Geometry check sheet. Reference: the model listing, model coordinates, mm. A direction names the side the tool comes from. Coordinates: 2 decimals unless noted, no trailing zeros. Write each loop counter-clockwise with the first axis right and the second up, starting at its lowest first coordinate (ties: lowest second). Pieces come first, ordered by that corner, then holes. Notation, with made-up numbers: (-3.5, 70) - (18.5, 70) arc R21 cw to (18.5, 78) - close; hole circle Ø1 at (82.5, 45.5). An arc over 180 degrees is marked (long way). Answer as a JSON object with one key per item and string values. Group by question number.
from build123d import *

# Parameters (mm, degrees)
SKETCH1_W           = 20
SKETCH1_H           = 20
SKETCH1_R           = 6
BOSS_EXTRUDE1_DEPTH = 5


with BuildPart() as part:
    # Sketch1 → Boss-Extrude1 (new body)
    # profile 1 of 3: a face of its own
    with BuildSketch(Plane.XY):
        Rectangle(SKETCH1_W, SKETCH1_H)
        Circle(SKETCH1_R, mode=Mode.SUBTRACT)
    # profile 2 of 3: a face of its own
    with BuildSketch(Plane.XY):
        with BuildLine():
            ThreePointArc((3.31662479, 5), (0, 6), (-3.31662479, 5))
            Line((-3.31662479, 5), (3.31662479, 5))
        make_face()
    # profile 3 of 3: a face of its own
    with BuildSketch(Plane.XY):
        with BuildLine():
            Line((3.31662479, -5), (-3.31662479, -5))
            ThreePointArc((-3.31662479, -5), (0, -6), (3.31662479, -5))
        make_face()
    extrude(amount=BOSS_EXTRUDE1_DEPTH)


solid = part.part
(1) Section check C-C (x = -5.25). Record the cut outline in (y, z).
(2) Material ranges on L1, parallel to Y at x = -1.75, z = 1.6; L2, parallel to Y at x = -5.5, z = 0.5; L3, parallel to X at y = 1, z = 3.8, recorded low to high. Write a range as [from, to].
(3) Gauge pin test, flat end, axial feed: pin 1 (4 mm diameter, centred on x = 6.5, y = -2.5, fed in from -Z). Record the tip position at first contact, or that the pin passes through.
(4) Section check B-B (y = 0.5). Record the cut outline in (x, z).
(5) Draft check along X on faces 1 (the face through (0, -5, 2)), 2 (the face through (10, 0, 2)), 3 (the face through (4, 5, 0)). Enter one of: +X half, -X half, draft (parallel to the pull), parting line (faces both ways), or undercut.
(6) Set-up check for faces 4 (the face through (4, 5, 5)), 5 (the face through (-6, 0, 2)): record each of +Z, -Z, +X, -X, +Y, -Y from which the full face is reachable in a straight line by a thin tool's end or side.
(7) Section check A-A (z = 2.8). Record the cut outline in (x, y), and give its area (3 significant figures).
Conclusion:
{
 "1": {"outline": "(-10, 0) - (-2.9, 0) - (-2.9, 5) - (-10, 5) - close; (2.9, 0) - (10, 0) - (10, 5) - (2.9, 5) - close"},
 "2": {"L1": "y = [-10, -5], [5, 10]", "L2": "y = [-10, -2.4], [2.4, 10]", "L3": "x = [-10, -5.92], [5.92, 10]"},
 "3": {"pin 1": "stops at z = 0"},
 "4": {"outline": "(-10, 0) - (-5.98, 0) - (-5.98, 5) - (-10, 5) - close; (5.98, 0) - (10, 0) - (10, 5) - (5.98, 5) - close"},
 "5": {"face 1": "undercut", "face 2": "+X half", "face 3": "draft"},
 "6": {"face 4": "+Z, +X, -X, +Y, -Y", "face 5": "+Z, -Z"},
 "7": {"outline": "(-10, -10) - (10, -10) - (10, 10) - (-10, 10) - close; hole (-3.32, -5) - (3.32, -5) arc R6 ccw to (3.32, 5) - (-3.32, 5) arc R6 ccw to start", "area": "296 mm^2"}
}
